Read the model definition and answer for the solid it produces. Units are mm, in the model's axes. Coordinates: 2 decimals unless noted, no trailing zeros. Loops run counter-clockwise (first coordinate to the right, second up) from the corner with the lowest first, then second, coordinate; pieces in that order, holes last. Notation, with made-up numbers: (1, 32) -> (32, 32) arc R20 ccw to (32, 55) -> close; hole circle Ø6 at (67, 7). An arc over 180 degrees is marked (long way). Answer as a JSON object with one key per item and string values. Group by question number.
1) Determine the mould class of faces 1 (the face through (-72.74, 2.85, 2.53)), 2 (the face through (-3, 1, 0)) for opening direction X: released by +X, released by -X, zero draft, split by the parting line, or undercut.
2) Flat-ended cylindrical pins translate along their axes: P1, Ø1.5, axis at y = -22.5, z = 2, coming from the +X side; P2, Ø1.5, axis at y = 33.5, z = 2.5, coming from the -X side; P3, Ø1.5, axis at x = 167, y = -36, coming from the -Z side. Find the tip coordinate at first contact, or state that the pin passes through.
3) Consider probe 1 along Y at (x, z) = (-90, 1.7); probe 2 along X at (y, z) = (-24, 2.75); probe 3 along X at (y, z) = (7, 2.8). Determine where each line is inside the solid, lowest interval first. Write a range as [from, to].
4) Section C-C, the plane z = 0.9 is taken. Count the separate pieces of the cut face and the enclosed holes in it, plus the area to 3 significant figures.
5) Section B-B, the plane x = 90 is taken. Give the vertices of the cut face in (y, z), plus the area to 3 significant figures.
6) Section A-A, the plane y = -26 is taken. Give the vertices of the cut face in (x, z), plus the area to 3 significant figures.
from build123d import *

# Parameters (mm, degrees)
SKETCH1_W                = 452
SKETCH1_H                = 90
BOSS_EXTRUDE1_DEPTH      = 5
SKETCH2_W                = 5.2
SKETCH2_H                = 25.2
CUT_EXTRUDE1_DEPTH       = 231.490780727
SKETCH4_W                = 5
SKETCH4_H                = 30
CUT_EXTRUDE5_DEPTH       = 5
SKETCH7_R                = 1
CUT_EXTRUDE6_DEPTH       = 231.490780727
FILLET4_R                = 1
SKETCH8_W                = 20.2
SKETCH8_H                = 10
CUT_EXTRUDE7_DEPTH       = 10
SKETCH9_W                = 20.2
SKETCH9_H                = 10
CUT_EXTRUDE8_DEPTH       = 300
MIRROR5_COPY_1_SKETCH_W  = 20.2
MIRROR5_COPY_1_SKETCH_H  = 10
MIRROR5_COPY_1_DEPTH     = 10
SKETCH11_R               = 4.25
CUT_EXTRUDE10_DEPTH      = 20
CUT_EXTRUDE11_DEPTH      = 30
CUT_EXTRUDE11_DEPTH_BACK = 600
SKETCH12_R               = 4.25


with BuildPart() as part:
    # Sketch1 → Boss-Extrude1 (new body)
    with BuildSketch(Plane.XY):
        Rectangle(SKETCH1_W, SKETCH1_H)
    extrude(amount=BOSS_EXTRUDE1_DEPTH)

    # Sketch2 → Cut-Extrude1 (cut, through all)
    with BuildSketch(Plane.XY.offset(5)):
        with Locations((0, 17.4)):
            Rectangle(SKETCH2_W, SKETCH2_H)
        with Locations((0, -17.4)):
            Rectangle(SKETCH2_W, SKETCH2_H)
    extrude(amount=-CUT_EXTRUDE1_DEPTH, mode=Mode.SUBTRACT)

    # Sketch4 → Cut-Extrude5 (cut)
    with BuildSketch(Plane.ZY.offset(226)):
        with Locations((2.5, 25)):
            Rectangle(SKETCH4_W, SKETCH4_H)
        with Locations((2.5, -25)):
            Rectangle(SKETCH4_W, SKETCH4_H)
    cut_extrude5 = extrude(amount=-CUT_EXTRUDE5_DEPTH, mode=Mode.SUBTRACT)

    # Mirror2: Cut-Extrude5 across plane
    add(cut_extrude5.mirror(Plane(origin=(0, 0, 0), x_dir=(0, 0, 1), z_dir=(1, 0, 0))), mode=Mode.SUBTRACT)

    # Sketch7 → Cut-Extrude6 (cut, through all)
    with BuildSketch(Plane.XY.offset(5)):
        with Locations((-221, 39)):
            Circle(SKETCH7_R)
        with Locations((-221, 11)):
            Circle(SKETCH7_R)
        with Locations((-221, -11)):
            Circle(SKETCH7_R)
        with Locations((-221, -39)):
            Circle(SKETCH7_R)
        with Locations((221, -39)):
            Circle(SKETCH7_R)
        with Locations((221, -11)):
            Circle(SKETCH7_R)
        with Locations((221, 11)):
            Circle(SKETCH7_R)
        with Locations((221, 39)):
            Circle(SKETCH7_R)
    extrude(amount=-CUT_EXTRUDE6_DEPTH, mode=Mode.SUBTRACT)

    # Fillet4
    fillet4_edges = [part.edges().sort_by_distance(p)[0] for p in [
        (221, 38, 2.5),
        (221, 12, 2.5),
        (221, -12, 2.5),
        (221, -38, 2.5),
        (-221, 38, 2.5),
        (-221, 12, 2.5),
        (-221, -38, 2.5),
        (-221, -12, 2.5),
        (-226, 10, 2.5),
        (-226, 40, 2.5),
        (-226, -40, 2.5),
        (-226, -10, 2.5),
        (226, 10, 2.5),
        (226, 40, 2.5),
        (226, -40, 2.5),
        (226, -10, 2.5),
    ]]
    fillet(fillet4_edges, radius=FILLET4_R)

    # Sketch8 → Cut-Extrude7 (cut)
    with BuildSketch(Plane(origin=(0, -610.456150304, 0), x_dir=(-1, 0, 0), z_dir=(0, 0, -1))):
        with Locations((-196, 585.456150304)):
            Rectangle(SKETCH8_W, SKETCH8_H)
    cut_extrude7 = extrude(amount=-CUT_EXTRUDE7_DEPTH, mode=Mode.SUBTRACT)

    # Mirror3: Cut-Extrude7 across plane
    add(cut_extrude7.mirror(Plane(origin=(0, 0, 0), x_dir=(0, 0, 1), z_dir=(1, 0, 0))), mode=Mode.SUBTRACT)

    # Sketch9 → Cut-Extrude8 (cut)
    with BuildSketch(Plane(origin=(0, -610.456150304, -223.6), x_dir=(-1, 0, 0), z_dir=(0, 0, -1))):
        with Locations((27.5, 585.456150304)):
            Rectangle(SKETCH9_W, SKETCH9_H)
    cut_extrude8 = extrude(amount=-CUT_EXTRUDE8_DEPTH, mode=Mode.SUBTRACT)

    # Mirror4: Cut-Extrude8 across plane
    add(cut_extrude8.mirror(Plane(origin=(0, 0, 0), x_dir=(0, 0, 1), z_dir=(1, 0, 0))), mode=Mode.SUBTRACT)

    # Mirror5: Cut-Extrude7 across plane
    add(cut_extrude7.mirror(Plane.ZX.offset(3.5)), mode=Mode.SUBTRACT)

    # Mirror5 copy 1 sketch → Mirror5 copy 1 (cut)
    with BuildSketch(Plane(origin=(0, 617.456150304, 0), x_dir=(1, 0, 0), z_dir=(0, 0, -1))):
        with Locations((-196, 585.456150304)):
            Rectangle(MIRROR5_COPY_1_SKETCH_W, MIRROR5_COPY_1_SKETCH_H)
    extrude(amount=-MIRROR5_COPY_1_DEPTH, mode=Mode.SUBTRACT)

    # Sketch11 → Cut-Extrude10 (cut)
    with BuildSketch(Plane(origin=(-635.072358446, 447.165636604, -5), x_dir=(1, 0, 0), z_dir=(0, 0, -1))):
        with Locations(Location((545.072358446, 420.165636604, 0), (0, 0, 180))):
            Circle(SKETCH11_R)
        with Locations(Location((545.072358446, 465.165636604, 0), (0, 0, 180))):
            Circle(SKETCH11_R)
    cut_extrude10 = extrude(amount=-CUT_EXTRUDE10_DEPTH, mode=Mode.SUBTRACT)

    # Mirror6: Cut-Extrude10 across plane
    add(cut_extrude10.mirror(Plane(origin=(0, 0, 0), x_dir=(0, 0, 1), z_dir=(1, 0, 0))), mode=Mode.SUBTRACT)

    # Sketch12 → Cut-Extrude11 (cut, two sides: drawn at the far end of the back side and taken through both)
    with BuildSketch(Plane(origin=(537.523634505, -819.47709654, 0), x_dir=(-1, 0, 0), z_dir=(0, 0, -1)).offset(-CUT_EXTRUDE11_DEPTH_BACK)):
        with Locations((611.181518753, 826.47709654)):
            Circle(SKETCH12_R)
        with Locations((463.865750257, 826.47709654)):
            Circle(SKETCH12_R)
    extrude(amount=CUT_EXTRUDE11_DEPTH + CUT_EXTRUDE11_DEPTH_BACK, mode=Mode.SUBTRACT)


solid = part.part
Determined:
{
 "1": {"face 1": "undercut", "face 2": "zero draft"},
 "2": {"P1": "x = 221", "P2": "x = -221", "P3": "z = 0"},
 "3": {"probe 1": "[-45, -22.25], [-13.75, 22.75], [31.25, 45]", "probe 2": "[-221, -206.1], [-185.9, -37.6], [-17.4, -2.6], [2.6, 17.4], [37.6, 185.9], [206.1, 221]", "probe 3": "[-226, -77.91], [-69.41, -2.6], [2.6, 69.41], [77.91, 226]"},
 "4": {"separate pieces": "1", "enclosed holes": "14", "area": "38,300 mm²"},
 "5": {"outline": "(-45, 0) -> (-22.25, 0) -> (-22.25, 5) -> (-45, 5) -> close; (-13.75, 0) -> (22.75, 0) -> (22.75, 5) -> (-13.75, 5) -> close; (31.25, 0) -> (45, 0) -> (45, 5) -> (31.25, 5) -> close", "area": "365 mm²"},
 "6": {"outline": "(-221, 0) -> (-206.1, 0) -> (-206.1, 5) -> (-221, 5) -> close; (-185.9, 0) -> (-37.6, 0) -> (-37.6, 5) -> (-185.9, 5) -> close; (-17.4, 0) -> (-2.6, 0) -> (-2.6, 5) -> (-17.4, 5) -> close; (2.6, 0) -> (17.4, 0) -> (17.4, 5) -> (2.6, 5) -> close; (37.6, 0) -> (185.9, 0) -> (185.9, 5) -> (37.6, 5) -> close; (206.1, 0) -> (221, 0) -> (221, 5) -> (206.1, 5) -> close", "area": "1,780 mm²"}
}
